```python
from build123d import *

# Parameters (mm, degrees)
SKETCH1_W               = 50.8
SKETCH1_H               = 25.4
SKETCH1_W_2             = 47.752
SKETCH1_H_2             = 22.352
EXTRUDE_THIN1_DEPTH     = 514.35
CUT_EXTRUDE1_DEPTH      = 518.47630139
CUT_EXTRUDE1_DEPTH_BACK = 518.47630139
SKETCH2_R               = 2.38125


with BuildPart() as part:
    # Sketch1 → Extrude-Thin1 (new body)
    with BuildSketch(Plane(origin=(0, 0, 0), x_dir=(1, 0, 0), z_dir=(0, 1, 0))):
        with Locations((-25.4, -12.7)):
            Rectangle(SKETCH1_W, SKETCH1_H)
        with Locations((-25.4, -12.7)):
            Rectangle(SKETCH1_W_2, SKETCH1_H_2, mode=Mode.SUBTRACT)
    extrude(amount=EXTRUDE_THIN1_DEPTH)

    # Sketch2 → Cut-Extrude1 (cut, two sides: drawn at the far end of the back side and taken through both)
    with BuildSketch(Plane.XY.offset(25.4).offset(-CUT_EXTRUDE1_DEPTH_BACK)):
        with Locations(Location((-38.1, 12.7, 0), (0, 0, 180))):
            Circle(SKETCH2_R)
        with Locations(Location((-25.4, 12.7, 0), (0, 0, 180))):
            Circle(SKETCH2_R)
        with Locations(Location((-12.7, 12.7, 0), (0, 0, 180))):
            Circle(SKETCH2_R)
        with Locations(Location((-38.1, 501.65, 0), (0, 0, 180))):
            Circle(SKETCH2_R)
        with Locations(Location((-25.4, 501.65, 0), (0, 0, 180))):
            Circle(SKETCH2_R)
        with Locations(Location((-12.7, 501.65, 0), (0, 0, 180))):
            Circle(SKETCH2_R)
    extrude(amount=CUT_EXTRUDE1_DEPTH + CUT_EXTRUDE1_DEPTH_BACK, mode=Mode.SUBTRACT)


solid = part.part
```
CAD build for the part. Positions are in the model's coordinates, mm. A direction names the side the tool comes from. Coordinates: 2 decimals unless noted, no trailing zeros. Write each loop counter-clockwise with the first axis right and the second up, starting at its lowest first coordinate (ties: lowest second). Pieces come first, ordered by that corner, then holes. Notation, with made-up numbers: (-34, 60) -> (8, 60) arc R26 ccw to (8, 83) -> close; hole circle Ø9 at (-17, 32). An arc over 180 degrees is marked (long way). Return JSON: item names as keys, results as strings. Group by question number.
Q1. Cut at A-A, the plane y = 420. Give the cut face in (x, z), then the cut area to 3 significant figures.
Q2. Pull direction X, two halves, no side cores. Call faces 1 (the face through (-1.524, 254, 13)), 2 (the face through (-26, 0, 25)), 3 (the face through (-26, 254, 1.524)), 4 (the face through (-50.8, 254, 13)): released by +X, released by -X, zero draft, split by the parting line, or undercut.
Q3. Drill centre lines: line 1 (Y direction, x = -25.4, z = 1.05); line 2 (X direction, y = 501.65, z = 1.15); line 3 (Z direction, x = -6, y = 84.5). Where is each one in solid material? Low to high.
Q4. Flat gauge pin, fed straight in: pin 1 (6 mm diameter, centred on x = -38.1, y = 501.65, fed in from -Z). Where does the tip first touch, or does it go through?
Q5. Which spindle directions (+Z, -Z, +X, -X, +Y, -Y) get a long thin tool onto all of the face, cutting with end or side? Do faces 5 (the face through (-26, 254, 23.876)), 6 (the face through (0, 254, 13)). Say none if no direction does.
Q6. Cut at B-B, the plane z = 13.5. Give the cut face in (x, y), then the cut area to 3 significant figures.
Returned:
{
 "1": {"outline": "(-50.8, 0) -> (0, 0) -> (0, 25.4) -> (-50.8, 25.4) -> close; hole (-49.28, 1.52) -> (-1.52, 1.52) -> (-1.52, 23.88) -> (-49.28, 23.88) -> close", "area": "223 mm2"},
 "2": {"face 1": "undercut", "face 2": "zero draft", "face 3": "undercut", "face 4": "released by -X"},
 "3": {"line 1": "y = 0 to 10.32, 15.08 to 499.27, 504.03 to 514.35", "line 2": "x = -50.8 to -40.48, -35.72 to -27.78, -23.02 to -15.08, -10.32 to 0", "line 3": "z = 0 to 1.52, 23.88 to 25.4"},
 "4": {"pin 1": "stops at z = 0"},
 "5": {"face 5": "+Y, -Y", "face 6": "+Z, -Z, +X, +Y, -Y"},
 "6": {"outline": "(-50.8, 0) -> (-49.28, 0) -> (-49.28, 514.35) -> (-50.8, 514.35) -> close; (-1.52, 0) -> (0, 0) -> (0, 514.35) -> (-1.52, 514.35) -> close", "area": "1,570 mm2"}
}
